from build123d import *

# Parameters (mm, degrees)
SKETCH_1_R      = 14.9225
EXTRUDE_1_DEPTH = 22


with BuildPart() as part:
    # Эскиз1 → Бобышка-Вытянуть1 (new body)
    with BuildSketch(Plane.XY):
        with Locations((0.26749168, -0.40123752)):
            Circle(SKETCH_1_R)
        with BuildLine():
            Line((9.068894716, -4.016260259), (9.770849808, -4.421534221))
            ThreePointArc((9.770849808, -4.421534221), (10.58624167, -0.401237512), (9.770849811, 3.619059197))
            Line((9.770849811, 3.619059197), (9.068894716, 3.213785234))
            Line((9.068894716, 3.213785234), (7.798894722, 5.413489748))
            Line((7.798894722, 5.413489748), (8.500849816, 5.81876371))
            ThreePointArc((8.500849816, 5.81876371), (5.426866673, 8.535062117), (1.537491677, 9.839060403))
            Line((1.537491677, 9.839060403), (1.537491677, 9.02851248))
            Line((1.537491677, 9.02851248), (-1.002508323, 9.02851248))
            Line((-1.002508323, 9.02851248), (-1.002508323, 9.839060408))
            ThreePointArc((-1.002508323, 9.839060408), (-4.891883323, 8.535062121), (-7.965866467, 5.818763712))
            Line((-7.965866467, 5.818763712), (-7.26391137, 5.413489747))
            Line((-7.26391137, 5.413489747), (-8.533911366, 3.213785229))
            Line((-8.533911366, 3.213785229), (-9.235866458, 3.61905919))
            ThreePointArc((-9.235866458, 3.61905919), (-10.05125832, -0.401237517), (-9.235866461, -4.421534225))
            Line((-9.235866461, -4.421534225), (-8.533911367, -4.016260262))
            Line((-8.533911367, -4.016260262), (-7.263911371, -6.215964781))
            Line((-7.263911371, -6.215964781), (-7.965866465, -6.621238743))
            ThreePointArc((-7.965866465, -6.621238743), (-4.891883323, -9.337537149), (-1.002508328, -10.641535436))
            Line((-1.002508328, -10.641535436), (-1.002508328, -9.830987512))
            Line((-1.002508328, -9.830987512), (1.537491672, -9.830987512))
            Line((1.537491672, -9.830987512), (1.537491672, -10.641535441))
            ThreePointArc((1.537491672, -10.641535441), (5.426866673, -9.337537153), (8.500849818, -6.621238742))
            Line((8.500849818, -6.621238742), (7.79889472, -6.215964777))
            Line((7.79889472, -6.215964777), (9.068894716, -4.016260259))
        make_face(mode=Mode.SUBTRACT)
    extrude(amount=EXTRUDE_1_DEPTH)


solid = part.part
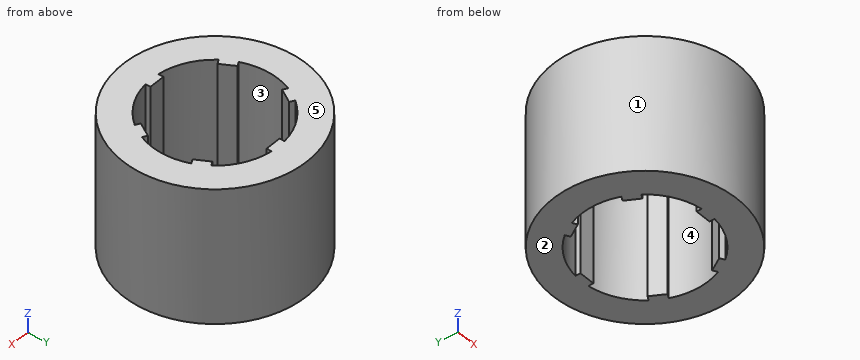
Here's how the part is built. I have some questions about the finished solid (model axes, mm). Face numbers are marked on the shaded views. A direction names the side the tool comes from. Coordinates: 2 decimals unless noted, no trailing zeros. Loops run counter-clockwise (first coordinate to the right, second up) from the corner with the lowest first, then second, coordinate; pieces in that order, holes last.
1. If we mould it in two halves opening along X, with no side actions, what happens to the marked faces 1, 2 and 3? For each: pulls with the +X half, pulls with the -X half, needs draft (parallel to the pull), parting line crosses it, or undercut.
2. Imagine slicing it at A-A, the plane y = -10.25. Please give me the cut outline in (x, z), and give its area (3 significant figures).
3. Imagine slicing it at D-D, the plane z = 15.75. Please give me the cut outline in (x, y) (1 decimal), and give its area (3 significant figures).
4. I need wall thicknesses on L1, parallel to Y at x = 0.25, z = 6.5; L2, parallel to X at y = 8.5, z = 6.25; L3, parallel to Y at x = -2, z = 17. Which ranges of each line are inside material? Lowest first, please.
5. Imagine slicing it at B-B, the plane x = 5. Please give me the cut outline in (y, z), and give its area (3 significant figures).
6. Imagine slicing it at C-C, the plane y = 4. Please give me the cut outline in (x, z), and give its area (3 significant figures).
7. For P1, Ø1, axis at y = 7.5, z = 13.5, coming from the -X side; P2, Ø1.5, axis at x = 2, z = 10, coming from the -Y side; P3, Ø0.6, axis at y = -10.5, z = 15.5, coming from the +X side; P4, Ø10, axis at x = -5, y = 6.5, coming from the -Z side, each with a flat end and sliding along its axis, tell me the tip position at first contact or that it passes through.
8. For the marked faces 4 and 5, which set-ups out of +Z, -Z, +X, -X, +Y, -Y let a thin tool reach every point of the face, with its end or its side?
Taken from the geometry:
1. face 1: parting line crosses it
1. face 2: needs draft
1. face 3: undercut
2. outline: (-10.94, 0) - (-2.81, 0) - (-2.81, 22) - (-10.94, 22) - close; (-1, 0) - (1.54, 0) - (1.54, 22) - (-1, 22) - close; (3.35, 0) - (11.48, 0) - (11.48, 22) - (3.35, 22) - close
2. area: 414 mm2
3. outline: circle Ø29.8 at (0.3, -0.4); hole (-9.2, -4.4) - (-8.5, -4) - (-7.3, -6.2) - (-8, -6.6) arc R10.3 ccw to (-1, -10.6) - (-1, -9.8) - (1.5, -9.8) - (1.5, -10.6) arc R10.3 ccw to (8.5, -6.6) - (7.8, -6.2) - (9.1, -4) - (9.8, -4.4) arc R10.3 ccw to (9.8, 3.6) - (9.1, 3.2) - (7.8, 5.4) - (8.5, 5.8) arc R10.3 ccw to (1.5, 9.8) - (1.5, 9) - (-1, 9) - (-1, 9.8) arc R10.3 ccw to (-8, 5.8) - (-7.3, 5.4) - (-8.5, 3.2) - (-9.2, 3.6) arc R10.3 ccw to start
3. area: 378 mm2
4. L1: y = -15.32 to -9.83, 9.03 to 14.52
4. L2: x = -11.71 to -4.95, 5.49 to 12.24
4. L3: y = -15.15 to -10.47, 9.67 to 14.35
5. outline: (-14.55, 0) - (-9.57, 0) - (-9.57, 22) - (-14.55, 22) - close; (8.77, 0) - (13.75, 0) - (13.75, 22) - (8.77, 22) - close
5. area: 219 mm2
6. outline: (-13.99, 0) - (-8.08, 0) - (-8.08, 22) - (-13.99, 22) - close; (8.61, 0) - (14.53, 0) - (14.53, 22) - (8.61, 22) - close
6. area: 260 mm2
7. P1: stops at x = -12.69
7. P2: stops at y = -15.29
7. P3: stops at x = 11.52
7. P4: stops at z = 0
8. face 4: +Z, -Z
8. face 5: +Z, +X, -X, +Y, -Y
